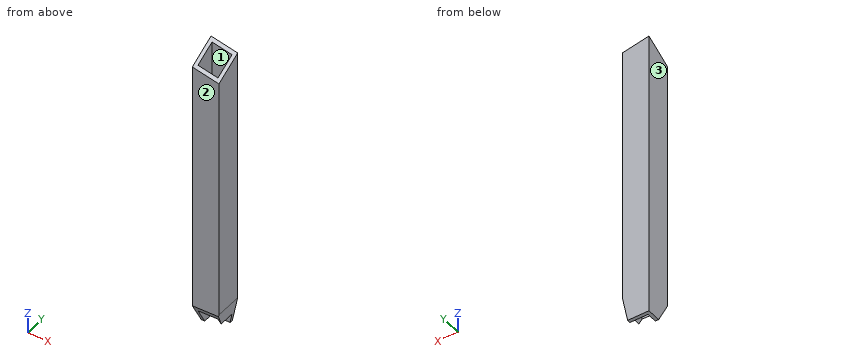
```python
from build123d import *

# Parameters (mm, degrees)
BOSS_EXTRUDE1_DEPTH      = 139.7
BOSS_EXTRUDE1_DEPTH_BACK = 139.7
SKETCH3_W                = 25.4
SKETCH3_H                = 25.4
SKETCH3_W_2              = 19.05
SKETCH3_H_2              = 19.05


with BuildPart() as part:
    # Sketch3 → Boss-Extrude1 (new, two sides: drawn at the far end of the back side and taken through both)
    with BuildSketch(Plane.XY.offset(-BOSS_EXTRUDE1_DEPTH_BACK)):
        Rectangle(SKETCH3_W, SKETCH3_H)
        Rectangle(SKETCH3_W_2, SKETCH3_H_2, mode=Mode.SUBTRACT)
    extrude(amount=BOSS_EXTRUDE1_DEPTH + BOSS_EXTRUDE1_DEPTH_BACK)

    # SurfaceCut2
    split(bisect_by=Plane(origin=(19.203056865, -53.641884581, 96.452303833), x_dir=(0.9807512157806098, 0, -0.1952614983678451), z_dir=(0.17141995510435715, -0.47884508758591265, 0.8610009181684186)), keep=Keep.BOTTOM)

    # SurfaceCut4
    split(bisect_by=Plane(origin=(34.104573835, 0, -6.790009618), x_dir=(0, 1, 0), z_dir=(0.9807512157806096, 0, -0.19526149836784543)), keep=Keep.BOTTOM)

    # SurfaceCut6
    split(bisect_by=Plane(origin=(1.132350751, -58.878507635, -32.094967554), x_dir=(0.9998151166046026, 0.01922843230544169, 0), z_dir=(0.01688375098917382, -0.8778994145657232, -0.478547340247228)), keep=Keep.BOTTOM)


solid = part.part
```
Check sheet for the modelled part. Datum: model origin and axes. Units: mm. Face numbers are marked on the shaded views. Give positions to 0.01 mm unless a question says otherwise; leave off trailing zeros. Write each loop counter-clockwise with the first axis right and the second up, starting at its lowest first coordinate (ties: lowest second). Pieces come first, ordered by that corner, then holes.
Item 1: Cross-section at C-C (z = 113). Enter the section's corners in (x, y) (3 decimals).
Item 2: Cross-section at B-B (x = 5). Enter the section's corners in (y, z) (3 decimals).
Item 3: Scan lines: L1, parallel to X at y = 6.5, z = 110 (3 decimals); L2, parallel to Z at x = 3, y = -11.25. Record each from-to range of solid material in increasing order.
Item 4: Draft check along X on the marked faces 1, 2 and 3. Enter one of: released by +X, released by -X, zero draft, split by the parting line, or undercut.
Item 5: Cross-section at A-A (y = 4). Enter the section's corners in (x, z) (1 decimal).
Item 6: Gauge pin test, flat ends, axial feed: pin 1 (4 mm diameter, centred on x = -8.5, y = -9, fed in from +Z); pin 2 (4 mm diameter, centred on x = 8, y = 2, fed in from +Z); pin 3 (6 mm diameter, centred on x = 10, y = 10, fed in from +Z). Record the tip position at first contact, or that the pin passes through.
Report:
1. outline: (-12.7, -12.7) - (12.7, -12.7) - (12.7, 12.7) - (-12.7, 12.7) - close; hole (-9.525, -9.525) - (9.525, -9.525) - (9.525, 9.525) - (-9.525, 9.525) - close
2. outline: (-12.7, -116.673) - (-9.525, -122.498) - (-9.525, 123.816) - (-12.7, 122.05) - close; (9.525, -139.7) - (12.7, -139.7) - (12.7, 136.176) - (9.525, 134.41) - close
3. L1: x = -12.7 to -9.525, 9.525 to 12.7
3. L2: z = -119.4 to 123.25
4. face 1: undercut
4. face 2: zero draft
4. face 3: released by -X
5. outline: (-12.7, -139.7) - (-9.5, -139.7) - (-9.5, 134.2) - (-12.7, 134.9) - close; (9.5, -130.2) - (12.7, -114.3) - (12.7, 129.8) - (9.5, 130.4) - close
6. pin 1: stops at z = 127.95
6. pin 2: stops at z = 130.04
6. pin 3: stops at z = 135.44
